```python
from build123d import *

# Parameters (mm, degrees)
SKETCH1_R           = 9.25
SKETCH1_R_2         = 4
BOSS_EXTRUDE1_DEPTH = 6.4
SKETCH2_R           = 8.35
CUT_EXTRUDE1_DEPTH  = 1.85
FILLET1_R           = 1.75
SKETCH3_R           = 1
CUT_EXTRUDE2_DEPTH  = 4.55
CUT_EXTRUDE2_TAPER  = 5
CIRPATTERN1_COUNT   = 13


with BuildPart() as part:
    # Sketch1 → Boss-Extrude1 (new body)
    with BuildSketch(Plane(origin=(0, 0, 0), x_dir=(1, 0, 0), z_dir=(0, 1, 0))):
        Circle(SKETCH1_R)
        Circle(SKETCH1_R_2, mode=Mode.SUBTRACT)
    extrude(amount=BOSS_EXTRUDE1_DEPTH)

    # Sketch2 → Cut-Extrude1 (cut)
    with BuildSketch(Plane(origin=(0, 6.4, 0), x_dir=(1, 0, 0), z_dir=(0, 1, 0))):
        Circle(SKETCH2_R)
    extrude(amount=-CUT_EXTRUDE1_DEPTH, mode=Mode.SUBTRACT)

    # Fillet1
    fillet1_edges = [part.edges().sort_by_distance(p)[0] for p in [
        (-8.35, 4.55, 0),
    ]]
    fillet(fillet1_edges, radius=FILLET1_R)

    # Sketch3 → Cut-Extrude2 (cut)
    with BuildSketch(Plane(origin=(0, 4.55, 0), x_dir=(1, 0, 0), z_dir=(0, 1, 0))):
        with Locations((0, -5.5)):
            Circle(SKETCH3_R)
    cut_extrude2 = extrude(amount=-CUT_EXTRUDE2_DEPTH, taper=CUT_EXTRUDE2_TAPER, mode=Mode.SUBTRACT)

    # CirPattern1: Cut-Extrude2 ×13 about axis
    cirpattern1_axis = Axis((0, 0, 0), (0, 1, 0))
    for i in range(1, CIRPATTERN1_COUNT):
        add(cut_extrude2.rotate(cirpattern1_axis, i * 360 / CIRPATTERN1_COUNT), mode=Mode.SUBTRACT)


solid = part.part
```
Can you work these out from the model? Positions are in its coordinate system, mm. A direction names the side the tool comes from. Coordinates: 2 decimals unless noted, no trailing zeros. Loops run counter-clockwise (first coordinate to the right, second up) from the corner with the lowest first, then second, coordinate; pieces in that order, holes last. Notation, with made-up numbers: M 10.5,-2 L 19.5,-2 A22 ccw 19.5,20 Z; hole C -35.75,70 d10. An arc over 180 degrees is marked long. Put each result on its own line as item: value. Start each with the question number.
(1) Will these pins go through, and if not, where does the flat tip stop? pin 1 Ø4 at (x, z) = (4, -0.5) entering from +Y; pin 2 Ø1.5 at (y, z) = (1.5, 4.5) entering from +X.
(2) Imagine slicing it at A-A on y = 3.75. Give the number of separate pieces and of enclosed holes in the cut face, and give its area (3 significant figures).
(3) Imagine slicing it at B-B on x = 0. List the corners of the cut face in (y, z) for me, and give its area (3 significant figures).
(4) I need wall thicknesses on probe 1 along Z at (x, y) = (0, 6.35); probe 2 along X at (y, z) = (3, 3.25); probe 3 along X at (y, z) = (3.5, 0). Which ranges of each line are inside material? Lowest first, please.
(5) We'd pull the mould along X, two halves only. Please class faces 3 (the face through (-4.2, 0, -0.1)), 4 (the face through (-2.01, 3.16, 9.03)), 5 (the face through (-1.84, 2.24, -5.94)), 6 (the face through (4.84, 2.24, 0.16)): +X half, -X half, draft (parallel to the pull), parting line (faces both ways), or undercut.
(6) Which directions (+Z, -Z, +X, -X, +Y, -Y) give clear straight access to the entire face, cutting with the end or side of a thin tool? Please do faces 1 (the face through (-5, 6.4, -7)), 2 (the face through (3, 4.55, -3)).
Worked answers:
1. pin 1: stops at y = 4.55
1. pin 2: stops at x = 8.46
2. separate pieces: 1
2. enclosed holes: 14
2. area: 183 mm2
3. outline: M 0,-9.25 L 6.4,-9.25 L 6.4,-8.35 L 6.3,-8.35 A1.75 cw 4.55,-6.6 L 4.55,-4 L 0,-4 Z; M 0,4 L 4.55,4 L 4.55,4.5 L 0,4.9 Z; M 0,6.1 L 4.55,6.5 L 4.55,6.6 A1.75 cw 6.3,8.35 L 6.4,8.35 L 6.4,9.25 L 0,9.25 Z
3. area: 45.1 mm2
4. probe 1: z = -9.25 to -8.35, 8.35 to 9.25
4. probe 2: x = -8.66 to -5.38, -3.67 to -2.33, 2.33 to 3.67, 5.38 to 8.66
4. probe 3: x = -9.25 to -6.08, -4.84 to -4, 4 to 4.84, 6.08 to 9.25
5. face 3: draft
5. face 4: parting line
5. face 5: undercut
5. face 6: undercut
6. face 1: +Z, -Z, +X, -X, +Y
6. face 2: +Y
